The listing builds one solid part. Answer for the finished solid, in the listing's coordinates (mm). Coordinates: 2 decimals unless noted, no trailing zeros. Order: outer loops, then holes, each group sorted by start corner. A loop starts at its lowest first (then second) coordinate and runs counter-clockwise, first axis right, second up. Notation, with made-up numbers: (54.5, 10) - (99.5, 10) arc R13 cw to (99.5, 19) - close; hole circle Ø7 at (35.25, -28). An arc over 180 degrees is marked (long way). Use one line per item in the form item = value. Start each with the question number.
Item 1: Section B-B, the plane z = 1106 is taken. Write down the section's boundary in (x, y).
Item 2: Consider line 1 along X through (y, z) = (17, 415); line 2 along X through (y, z) = (27.5, 124). Determine where each line is inside the solid, lowest interval first. Write a range as [from, to].
Item 3: Each of these flat-tipped pins is pushed along its axis until it touches: pin 1 Ø1.4 at (x, z) = (31, 644.5) entering from -Y; pin 2 Ø0.6 at (x, z) = (31, 646) entering from +Y. Where does it stop, or does it pass through?
Item 4: Section A-A, the plane x = 0 is taken. Write down the section's boundary in (y, z), and give its area (3 significant figures).
Item 5: Section C-C, the plane z = 539 is taken. Write down the section's boundary in (x, y), and give its area (3 significant figures).
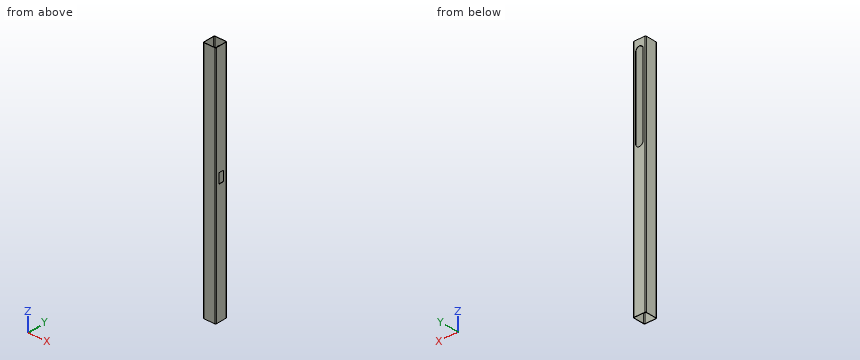
from build123d import *

# Parameters (mm, degrees)
F1_DEPTH = 1219.2
F3_DEPTH = 1.27
F5_DEPTH = 1.27


with BuildPart() as f1:
    # F0 (on Top) → F1 (new body)
    with BuildSketch(Plane.XY):
        with BuildLine():
            ThreePointArc((31.75, 27.94), (30.634077, 30.634077), (27.94, 31.75))
            Line((27.94, 31.75), (-27.94, 31.75))
            ThreePointArc((-27.94, 31.75), (-30.634077, 30.634077), (-31.75, 27.94))
            Line((-31.75, 27.94), (-31.75, -27.94))
            ThreePointArc((-31.75, -27.94), (-30.634077, -30.634077), (-27.94, -31.75))
            Line((-27.94, -31.75), (27.94, -31.75))
            ThreePointArc((27.94, -31.75), (30.634077, -30.634077), (31.75, -27.94))
            Line((31.75, -27.94), (31.75, 27.94))
        make_face()
        with BuildLine():
            Line((-26.67, 30.48), (26.67, 30.48))
            ThreePointArc((26.67, 30.48), (29.364077, 29.364077), (30.48, 26.67))
            Line((30.48, 26.67), (30.48, -26.67))
            ThreePointArc((30.48, -26.67), (29.364077, -29.364077), (26.67, -30.48))
            Line((26.67, -30.48), (-26.67, -30.48))
            ThreePointArc((-26.67, -30.48), (-29.364077, -29.364077), (-30.48, -26.67))
            Line((-30.48, -26.67), (-30.48, 26.67))
            ThreePointArc((-30.48, 26.67), (-29.364077, 29.364077), (-26.67, 30.48))
        make_face(mode=Mode.SUBTRACT)
    extrude(amount=F1_DEPTH)

    # F2 (on face) → F3 (cut, through all)
    with BuildSketch(Plane(origin=(0, 31.75, 0), x_dir=(-1, 0, 0), z_dir=(0, 1, 0))):
        with BuildLine():
            ThreePointArc((19.05, 1168.4), (0, 1187.45), (-19.05, 1168.4))
            Line((-19.05, 1168.4), (-19.05, 762))
            ThreePointArc((-19.05, 762), (0, 742.95), (19.05, 762))
            Line((19.05, 762), (19.05, 1168.4))
        make_face()
    extrude(amount=-F3_DEPTH, mode=Mode.SUBTRACT)

    # F4 (on face) → F5 (cut, through all)
    with BuildSketch(Plane.YZ.offset(31.75)):
        with BuildLine():
            ThreePointArc((12.7, 657.86), (11.956051, 659.656051), (10.16, 660.4))
            Line((10.16, 660.4), (-10.16, 660.4))
            ThreePointArc((-10.16, 660.4), (-11.956051, 659.656051), (-12.7, 657.86))
            Line((-12.7, 657.86), (-12.7, 612.14))
            ThreePointArc((-12.7, 612.14), (-11.956051, 610.343949), (-10.16, 609.6))
            Line((-10.16, 609.6), (10.16, 609.6))
            ThreePointArc((10.16, 609.6), (11.956051, 610.343949), (12.7, 612.14))
            Line((12.7, 612.14), (12.7, 657.86))
        make_face()
    extrude(amount=-F5_DEPTH, mode=Mode.SUBTRACT)


solid = f1.part
Response:
q1.outline = (-31.75, -27.94) arc R3.81 ccw to (-27.94, -31.75) - (27.94, -31.75) arc R3.81 ccw to (31.75, -27.94) - (31.75, 27.94) arc R3.81 ccw to (27.94, 31.75) - (19.05, 31.75) - (19.05, 30.48) - (26.67, 30.48) arc R3.81 cw to (30.48, 26.67) - (30.48, -26.67) arc R3.81 cw to (26.67, -30.48) - (-26.67, -30.48) arc R3.81 cw to (-30.48, -26.67) - (-30.48, 26.67) arc R3.81 cw to (-26.67, 30.48) - (-19.05, 30.48) - (-19.05, 31.75) - (-27.94, 31.75) arc R3.81 ccw to (-31.75, 27.94) - close
q2.line_1 = [-31.75, -30.48], [30.48, 31.75]
q2.line_2 = [-31.75, -30.39], [30.39, 31.75]
q3.pin_1 = -30.93
q3.pin_2 = 30.57
q4.outline = (-31.75, 0) - (-30.48, 0) - (-30.48, 1219.2) - (-31.75, 1219.2) - close; (30.48, 0) - (31.75, 0) - (31.75, 742.95) - (30.48, 742.95) - close; (30.48, 1187.45) - (31.75, 1187.45) - (31.75, 1219.2) - (30.48, 1219.2) - close
q4.area = 2,530 mm2
q5.outline = (-31.75, -27.94) arc R3.81 ccw to (-27.94, -31.75) - (27.94, -31.75) arc R3.81 ccw to (31.75, -27.94) - (31.75, 27.94) arc R3.81 ccw to (27.94, 31.75) - (-27.94, 31.75) arc R3.81 ccw to (-31.75, 27.94) - close; hole (-30.48, -26.67) arc R3.81 ccw to (-26.67, -30.48) - (26.67, -30.48) arc R3.81 ccw to (30.48, -26.67) - (30.48, 26.67) arc R3.81 ccw to (26.67, 30.48) - (-26.67, 30.48) arc R3.81 ccw to (-30.48, 26.67) - close
q5.area = 316 mm2
